Build history of the part. All positions in model axes, mm. A direction names the side the tool comes from. Round coordinates to 2 decimals unless told otherwise and drop trailing zeros. Order: outer loops, then holes, each group sorted by start corner. A loop starts at its lowest first (then second) coordinate and runs counter-clockwise, first axis right, second up. Notation, with made-up numbers: (-14, 3.5) -> (40, 3.5) arc R20 ccw to (40, 32.5) -> close; hole circle Ø3 at (4, 7.25). An arc over 180 degrees is marked (long way). Answer as a JSON object with one key per item and string values.
from build123d import *

# Parameters (mm, degrees)
BOSS_EXTRU_1_DEPTH = 5.5
ESQUISSE2_R        = 4
BOSS_EXTRU_2_DEPTH = 60


with BuildPart() as part:
    # Esquisse1 → Boss.-Extru.1 (new body)
    with BuildSketch(Plane(origin=(0, 0, 0), x_dir=(1, 0, 0), z_dir=(0, 1, 0))):
        Polygon((6.5, 3.75277675), (0, 7.505553499), (-6.5, 3.75277675), (-6.5, -3.75277675), (0, -7.505553499), (6.5, -3.75277675), align=None)
    extrude(amount=BOSS_EXTRU_1_DEPTH)

    # Esquisse2 → Boss.-Extru.2 (add)
    with BuildSketch(Plane(origin=(0, 0, 0), x_dir=(1, 0, 0), z_dir=(0, 1, 0))):
        with Locations(Location((0, 0, 0), (0, 0, 270))):
            Circle(ESQUISSE2_R)
    extrude(amount=-BOSS_EXTRU_2_DEPTH)


solid = part.part
1) Cut at D-D, the plane y = -37. Give the cut face in (x, z), plus the area to 3 significant figures.
Checked values:
{"outline": "circle Ø8 at (0, 0)", "area": "50.3 mm²"}
2) Cut at C-C, the plane x = -2.75. Give the cut face in (y, z), plus the area to 3 significant figures.
Checked values:
{"outline": "(-60, -2.9) -> (0, -2.9) -> (0, -5.92) -> (5.5, -5.92) -> (5.5, 5.92) -> (0, 5.92) -> (0, 2.9) -> (-60, 2.9) -> close", "area": "414 mm²"}
3) Cut at A-A, the plane z = 0. Give the cut face in (x, y).
Checked values:
{"outline": "(-6.5, 0) -> (-4, 0) -> (-4, -60) -> (4, -60) -> (4, 0) -> (6.5, 0) -> (6.5, 5.5) -> (-6.5, 5.5) -> close"}
4) Cut at B-B, the plane y = 1. Give the cut face in (x, z).
Checked values:
{"outline": "(-6.5, -3.75) -> (0, -7.51) -> (6.5, -3.75) -> (6.5, 3.75) -> (0, 7.51) -> (-6.5, 3.75) -> close"}
5) Flat gauge pins, fed straight in: pin 1 Ø4 at (x, y) = (-3, -12) entering from -Z; pin 2 Ø1.5 at (y, z) = (-39, -1) entering from -X; pin 3 Ø3 at (x, y) = (0.5, -37) entering from -Z. Where does each tip first touch, or does it go through?
Checked values:
{"pin 1": "stops at z = -3.87", "pin 2": "stops at x = -3.99", "pin 3": "stops at z = -4"}
6) Which spindle directions (+Z, -Z, +X, -X, +Y, -Y) get a long thin tool onto all of the face, cutting with end or side? Do faces 1 (the face through (-3.905, -29.58, -0.867)), 2 (the face through (0, -60, 0)). Say none if no direction does.
Checked values:
{"face 1": "-Y", "face 2": "+Z, -Z, +X, -X, -Y"}
7) Probe L1, parallel to Y at x = -4.75, z = -1.25; L2, parallel to Z at x = 1, y = -15.5; L3, parallel to X at y = -11.5, z = 0. List the from-to ranges inside material, lowest first. Write a range as from..to.
Checked values:
{"L1": "y = 0..5.5", "L2": "z = -3.87..3.87", "L3": "x = -4..4"}
